from build123d import *

# Parameters (mm, degrees)
BOSS_EXTRUDE1_DEPTH  = 82.5
SKETCH2_R            = 2.5
BOSS_EXTRUDE2_DEPTH  = 3
FILLET1_R            = 1
FILLET1_OF_MIRROR1_R = 1
BOSS_EXTRUDE3_DEPTH  = 25
FILLET2_SIZE         = 2
FILLET3_R            = 0.5


with BuildPart() as part:
    # Sketch1 → Boss-Extrude1 (new, symmetric)
    with BuildSketch(Plane(origin=(679.474882377, 899.436301878, 1292.844863494), x_dir=(0, 0, -1), z_dir=(1, 0, 0))):
        with BuildLine():
            Line((-167.2, 0), (-167.2, 55))
            ThreePointArc((-167.2, 55), (-153.375440072, 88.375440072), (-120, 102.2))
            Line((-120, 102.2), (0, 102.2))
            Line((0, 102.2), (0, 100.2))
            Line((0, 100.2), (-120, 100.2))
            ThreePointArc((-120, 100.2), (-151.96122651, 86.96122651), (-165.2, 55))
            Line((-165.2, 55), (-165.2, 0))
            Line((-165.2, 0), (-167.2, 0))
        make_face()
    extrude(amount=BOSS_EXTRUDE1_DEPTH, both=True)

    # Sketch2 → Boss-Extrude2 (add)
    with BuildSketch(Plane(origin=(721.724882377, 0, 0), x_dir=(0, 0, -1), z_dir=(1, 0, 0))):
        with BuildLine():
            Line((-1292.844863494, 999.636301878), (-1287.549744281, 996.914228228))
            ThreePointArc((-1287.549744281, 996.914228228), (-1281.103673423, 999.921643269), (-1285.623100176, 1005.414471007))
            Line((-1285.623100176, 1005.414471007), (-1297.448447634, 1005.070743882))
            Line((-1297.448447634, 1005.070743882), (-1297.448447634, 1001.636301878))
            Line((-1297.448447634, 1001.636301878), (-1292.844863494, 1001.636301878))
            Line((-1292.844863494, 1001.636301878), (-1292.844863494, 999.636301878))
        make_face()
        with Locations((-1285.492353992, 1000.916370804)):
            Circle(SKETCH2_R, mode=Mode.SUBTRACT)
    boss_extrude2 = extrude(amount=BOSS_EXTRUDE2_DEPTH)

    # Fillet1
    fillet1_edges = [part.edges().sort_by_distance(p)[0] for p in [
        (724.724882377, 1000.636301878, 1292.844863494),
        (724.724882377, 1001.636301878, 1295.146655564),
        (721.724882377, 1000.636301878, 1292.844863494),
        (723.224882377, 1005.070743882, 1297.448447634),
        (721.724882377, 1001.636301878, 1295.146655564),
        (723.224882377, 1001.636301878, 1297.448447634),
    ]]
    fillet(fillet1_edges, radius=FILLET1_R)

    # Mirror1: Boss-Extrude2 across plane
    add(boss_extrude2.mirror(Plane(origin=(679.474882377, 0, 0), x_dir=(0, 0, 1), z_dir=(1, 0, 0))))

    # Fillet1 of Mirror1
    fillet1_of_mirror1_edges = [part.edges().sort_by_distance(p)[0] for p in [
        (634.224882377, 1000.636301878, 1292.844863494),
        (634.224882377, 1001.636301878, 1295.146655564),
        (637.224882377, 1000.636301878, 1292.844863494),
        (635.724882377, 1005.070743882, 1297.448447634),
        (637.224882377, 1001.636301878, 1295.146655564),
        (635.724882377, 1001.636301878, 1297.448447634),
    ]]
    fillet(fillet1_of_mirror1_edges, radius=FILLET1_OF_MIRROR1_R)

    # Sketch3 → Boss-Extrude3 (add, symmetric)
    with BuildSketch(Plane(origin=(679.474882377, 0, 0), x_dir=(0, 0, -1), z_dir=(1, 0, 0))):
        with BuildLine():
            Line((-1458.044863494, 907.760575274), (-1456.444863494, 907.760575274))
            ThreePointArc((-1456.444863494, 907.760575274), (-1455.591310103, 908.114128665), (-1455.944863494, 907.260575274))
            Line((-1455.944863494, 907.260575274), (-1455.944863494, 904.260575274))
            Line((-1455.944863494, 904.260575274), (-1453.944863494, 904.260575274))
            Line((-1453.944863494, 904.260575274), (-1453.944863494, 909.760575274))
            Line((-1453.944863494, 909.760575274), (-1458.044863494, 909.760575274))
            Line((-1458.044863494, 909.760575274), (-1458.044863494, 907.760575274))
        make_face()
    extrude(amount=BOSS_EXTRUDE3_DEPTH, both=True)

    # Fillet2
    # a fillet whose section is not a circle: 2 mm, written as the material it takes off along each edge
    with BuildSketch(Plane(origin=(649.474882377, 904.260575274, 1455.944863494), x_dir=(0, 1, 0), z_dir=(1, 0, 0))) as fillet2_piece_1:
        with BuildLine():
            Bezier((FILLET2_SIZE, 0), (0, 0), (0, -FILLET2_SIZE), weights=[1, 0.538461538, 1])
            Line((0, -FILLET2_SIZE), (0, 0))
            Line((0, 0), (FILLET2_SIZE, 0))
        make_face()
    extrude(amount=60, mode=Mode.SUBTRACT)

    # Fillet3
    fillet3_edges = [part.edges().sort_by_distance(p)[0] for p in [
        (654.474882377, 907.010575274, 1453.944863494),
        (654.474882377, 909.760575274, 1455.994863494),
        (654.474882377, 908.760575274, 1458.044863494),
        (704.474882377, 908.760575274, 1458.044863494),
        (704.474882377, 909.760575274, 1455.994863494),
        (704.474882377, 907.010575274, 1453.944863494),
        (679.474882377, 909.760575274, 1458.044863494),
        (679.474882377, 909.760575274, 1453.944863494),
    ]]
    fillet(fillet3_edges, radius=FILLET3_R)


solid = part.part
Design review of the part built by this model. Coordinates are the model's own, in mm. A direction names the side the tool comes from. Coordinates: 2 decimals unless noted, no trailing zeros. Order: outer loops, then holes, each group sorted by start corner. A loop starts at its lowest first (then second) coordinate and runs counter-clockwise, first axis right, second up. Notation, with made-up numbers: (-0.5, -39) -> (27.5, -39) arc R31 cw to (27.5, -9) -> close; hole circle Ø5 at (0.5, 87.25). An arc over 180 degrees is marked (long way). One line per item, written item: value.
1) Machinability: for faces 1 (the face through (637.225, 1002, 1289)), 2 (the face through (635.76, 998.29, 1290.23)), 3 (the face through (680, 907, 1453.945)), 4 (the face through (634.225, 1002, 1289)), which of the approach directions +Z, -Z, +X, -X, +Y, -Y give a long, thin tool a straight path to every point of the face, cutting with its end or side? Answer none if there is none.
Output values:
face 1: -Z, +Y
face 2: +X, -X, -Y
face 3: -Z, +X, -X, -Y
face 4: -Z, -X, +Y
2) Clearance check with flat-ended pins moving along their axes: P1, Ø5, axis at x = 643.5, y = 938.5, coming from the -Z side; P2, Ø6, axis at y = 1000.92, z = 1285.49, coming from the +X side; P3, Ø1.5, axis at x = 628.5, z = 1424.5, coming from the +Y side. State where each tip first meets the part, or that it passes through.
Output values:
P1: stops at z = 1458.04
P2: stops at x = 724.72
P3: stops at y = 1000.36
3) We need section C-C, the plane y = 976. Give the boundary of the cut face in (x, z), then the cut area to 3 significant figures.
Output values:
outline: (596.97, 1452.57) -> (761.97, 1452.57) -> (761.97, 1454.83) -> (596.97, 1454.83) -> close
area: 373 mm2
4) To check wall thickness, follow probe 1 along Y at (x, z) = (627.5, 1410.5); probe 2 along Z at (x, y) = (671.5, 933); probe 3 along Z at (x, y) = (641, 963.5). State the ranges of each line that lie inside material, in increasing order. Write a range as [from, to].
Output values:
probe 1: y = [999.64, 1001.64]
probe 2: z = [1458.04, 1460.04]
probe 3: z = [1457.13, 1459.17]
5) We need section A-A, the plane x = 629.5. Give the boundary of the cut face in (y, z), then the cut area to 3 significant figures.
Output values:
outline: (899.44, 1458.04) -> (954.44, 1458.04) arc R45.2 cw to (999.64, 1412.84) -> (999.64, 1292.84) -> (1001.64, 1292.84) -> (1001.64, 1412.84) arc R47.2 ccw to (954.44, 1460.04) -> (899.44, 1460.04) -> close
area: 495 mm2
6) Draft analysis for pull direction Z (two halves, no side actions). For faces 5 (the face through (596.975, 1000, 1376)), 6 (the face through (680.63, 987.44, 1446.59)), 7 (the face through (723.19, 998.29, 1290.23)), state which applies: +Z half, -Z half, draft (parallel to the pull), parting line (faces both ways), or undercut.
Output values:
face 5: draft
face 6: +Z half
face 7: undercut
7) We need section B-B, the plane z = 1335. Give the boundary of the cut face in (x, y).
Output values:
outline: (596.97, 999.64) -> (761.97, 999.64) -> (761.97, 1001.64) -> (596.97, 1001.64) -> close
